Verification items for the finished model (mm, model axes). A direction names the side the tool comes from. Give positions to 0.01 mm unless a question says otherwise; leave off trailing zeros. Loops run counter-clockwise (first coordinate to the right, second up) from the corner with the lowest first, then second, coordinate; pieces in that order, holes last. Notation, with made-up numbers: (72, 80.5) -> (98, 80.5) arc R8 ccw to (98, 86.5) -> close; hole circle Ø11 at (14.25, 25). An arc over 180 degrees is marked (long way). Use one line per item in the form item = value. Start each with the question number.
from build123d import *

# Parameters (mm, degrees)
SKETCH1_W           = 70
SKETCH1_H           = 50
BOSS_EXTRUDE1_DEPTH = 75
CUT_EXTRUDE1_REACH  = 98.695
SKETCH2_R           = 7.5
SKETCH2_R_2         = 13
SKETCH3_R           = 2.5
CUT_EXTRUDE2_DEPTH  = 20


with BuildPart() as part:
    # Sketch1 → Boss-Extrude1 (new body)
    with BuildSketch(Plane.XY):
        Rectangle(SKETCH1_W, SKETCH1_H)
    extrude(amount=BOSS_EXTRUDE1_DEPTH)

    # Sketch2 → Cut-Extrude1 (cut, up to next)
    with BuildSketch(Plane(origin=(0, 25, 0), x_dir=(1, 0, 0), z_dir=(0, 1, 0)), mode=Mode.PRIVATE) as cut_extrude1_sk1:
        with Locations(Location((22.75, -25, 0), (0, 0, 180))):
            Circle(SKETCH2_R)
    cut_extrude1_tool1 = extrude(cut_extrude1_sk1.sketch, amount=-CUT_EXTRUDE1_REACH, mode=Mode.PRIVATE) & part.part
    # Sketch2 → Cut-Extrude1 (cut, up to next)
    with BuildSketch(Plane(origin=(0, 25, 0), x_dir=(1, 0, 0), z_dir=(0, 1, 0)), mode=Mode.PRIVATE) as cut_extrude1_sk2:
        with Locations(Location((-15, -25, 0), (0, 0, 180))):
            Circle(SKETCH2_R_2)
    cut_extrude1_tool2 = extrude(cut_extrude1_sk2.sketch, amount=-CUT_EXTRUDE1_REACH, mode=Mode.PRIVATE) & part.part
    add(cut_extrude1_tool1.solids().sort_by_distance((22.75, 25, 25))[0], mode=Mode.SUBTRACT)
    add(cut_extrude1_tool2.solids().sort_by_distance((-15, 25, 25))[0], mode=Mode.SUBTRACT)

    # Sketch3 → Cut-Extrude2 (cut)
    with BuildSketch(Plane.XY.offset(75)):
        with Locations((0, -20)):
            Circle(SKETCH3_R)
        with Locations(Location((0, 20, 0), (0, 0, 180))):
            Circle(SKETCH3_R)
    extrude(amount=-CUT_EXTRUDE2_DEPTH, mode=Mode.SUBTRACT)


solid = part.part
Item 1: Draft check along X on faces 1 (the flat face through (35, 0, 37)), 2 (the flat face through (0, -20, 55)), 3 (the flat face through (0, -25, 37)), 4 (the flat face through (-35, 0, 37)). Enter one of: +X half, -X half, draft (parallel to the pull), parting line (faces both ways), or undercut.
Item 2: Sectioned sample at C-C, the plane y = -20. Enter the section's corners in (x, z).
Item 3: Tool access check on faces 5 (the cylindrical face through (28.278, 0.35, 30.069)), 6 (the cylindrical face through (0.33, 17.52, 65.14)). Record the directions out of +Z, -Z, +X, -X, +Y, -Y that give a thin tool (end or side, any length) a straight path to the whole face; none if there is none.
Item 4: Sectioned sample at D-D, the plane x = 0. Enter the section's corners in (y, z).
Item 5: Material ranges on line 1 (Y direction, x = 0, z = 63); line 2 (X direction, y = -8, z = 29.5); line 3 (Z direction, x = -15, y = -6), recorded low to high.
Item 6: Sectioned sample at A-A, the plane z = 25. Enter the section's corners in (x, y).
Item 7: Sectioned sample at B-B, the plane x = -15. Enter the section's corners in (y, z), and give its area (3 significant figures).
Item 8: Gauge pin test, flat end, axial feed: pin 1 Ø2.5 at (x, y) = (-1, 19.5) entering from +Z. Record the tip position at first contact, or that the pin passes through.
Outcome:
q1.face_1 = +X half
q1.face_2 = undercut
q1.face_3 = draft
q1.face_4 = -X half
q2.outline = (-35, 0) -> (35, 0) -> (35, 75) -> (2.5, 75) -> (2.5, 55) -> (-2.5, 55) -> (-2.5, 75) -> (-35, 75) -> close; hole circle Ø26 at (-15, 25); hole circle Ø15 at (22.75, 25)
q3.face_5 = +Y, -Y
q3.face_6 = +Z
q4.outline = (-25, 0) -> (25, 0) -> (25, 75) -> (22.5, 75) -> (22.5, 55) -> (17.5, 55) -> (17.5, 75) -> (-17.5, 75) -> (-17.5, 55) -> (-22.5, 55) -> (-22.5, 75) -> (-25, 75) -> close
q5.line_1 = -25 to -22.5, -17.5 to 17.5, 22.5 to 25
q5.line_2 = -35 to -27.2, -2.8 to 16.75, 28.75 to 35
q5.line_3 = 0 to 12, 38 to 75
q6.outline = (-35, -25) -> (-28, -25) -> (-28, 25) -> (-35, 25) -> close; (-2, -25) -> (15.25, -25) -> (15.25, 25) -> (-2, 25) -> close; (30.25, -25) -> (35, -25) -> (35, 25) -> (30.25, 25) -> close
q7.outline = (-25, 0) -> (25, 0) -> (25, 12) -> (-25, 12) -> close; (-25, 38) -> (25, 38) -> (25, 75) -> (-25, 75) -> close
q7.area = 2,450 mm^2
q8.pin_1 = 55
